The listing builds one solid part. Answer for the finished solid, in the listing's coordinates (mm). A direction names the side the tool comes from. Coordinates: 2 decimals unless noted, no trailing zeros. Loops run counter-clockwise (first coordinate to the right, second up) from the corner with the lowest first, then second, coordinate; pieces in that order, holes last. Notation, with made-up numbers: (3.25, 81.5) - (7.25, 81.5) arc R21 cw to (7.25, 107.5) - close; hole circle Ø3 at (71.5, -23). An arc over 180 degrees is marked (long way). One line per question, with ' | ' between items.
from build123d import *

# Parameters (mm, degrees)
BOSS_EXTRUDE1_DEPTH  = 30
BOSS_EXTRUDE2_START  = -15
BOSS_EXTRUDE2_DEPTH  = 15
CUT_EXTRUDE1_START   = -15
CUT_EXTRUDE1_DEPTH   = 15
SKETCH5_R            = 1.5
CUT_EXTRUDE2_DEPTH   = 15
SKETCH6_R            = 3.1
CUT_EXTRUDE3_DEPTH   = 5
SKETCH7_R            = 1.5
CUT_EXTRUDE4_DEPTH   = 15
SKETCH8_R            = 3.1
CUT_EXTRUDE5_DEPTH   = 5
SKETCH11_R           = 7.5
CUT_EXTRUDE6_DEPTH   = 30
SKETCH12_R           = 11
CUT_EXTRUDE7_DEPTH   = 20
SKETCH13_R           = 4
BOSS_EXTRUDE3_DEPTH  = 20
FILLET1_R            = 2
FILLET1_OF_MIRROR1_R = 2
SKETCH14_R           = 4
CUT_EXTRUDE8_DEPTH   = 40


with BuildPart() as part:
    # Sketch2 → Boss-Extrude1 (new body)
    with BuildSketch(Plane(origin=(0, 0, 0), x_dir=(1, 0, 0), z_dir=(0, 1, 0))):
        with BuildLine():
            Line((-105, 0), (-80, 0))
            ThreePointArc((-80, 0), (0, -80), (80, 0))
            Line((80, 0), (105, 0))
            ThreePointArc((105, 0), (0, -105), (-105, 0))
        make_face()
    extrude(amount=BOSS_EXTRUDE1_DEPTH)

    # Sketch3 → Boss-Extrude2 (add)
    with BuildSketch(Plane(origin=(0, 30, 0), x_dir=(1, 0, 0), z_dir=(0, 1, 0)).offset(BOSS_EXTRUDE2_START)):
        with BuildLine():
            Line((-98.667725183, 35.912115049), (-75.175409663, 27.361611466))
            ThreePointArc((-75.175409663, 27.361611466), (-78.784620241, 13.891854213), (-80, 0))
            Line((-80, 0), (-105, 0))
            ThreePointArc((-105, 0), (-103.404814066, 18.233058655), (-98.667725183, 35.912115049))
        make_face()
    extrude(amount=BOSS_EXTRUDE2_DEPTH)

    # Sketch4 → Cut-Extrude1 (cut)
    with BuildSketch(Plane(origin=(0, 30, 0), x_dir=(1, 0, 0), z_dir=(0, 1, 0)).offset(CUT_EXTRUDE1_START)):
        with BuildLine():
            Line((80, 0), (105, 0))
            ThreePointArc((105, 0), (103.404814066, -18.233058655), (98.667725183, -35.912115049))
            Line((98.667725183, -35.912115049), (75.175409663, -27.361611466))
            ThreePointArc((75.175409663, -27.361611466), (78.784620241, -13.891854213), (80, 0))
        make_face()
    extrude(amount=CUT_EXTRUDE1_DEPTH, mode=Mode.SUBTRACT)

    # Sketch5 → Cut-Extrude2 (cut)
    with BuildSketch(Plane(origin=(0, 15, 0), x_dir=(1, 0, 0), z_dir=(0, 1, 0))):
        with Locations(Location((91.088089232, -16.1, 0), (0, 0, 270))):
            Circle(SKETCH5_R)
    extrude(amount=-CUT_EXTRUDE2_DEPTH, mode=Mode.SUBTRACT)

    # Sketch6 → Cut-Extrude3 (cut)
    with BuildSketch(Plane(origin=(0, 0, 0), x_dir=(-1, 0, 0), z_dir=(0, -1, 0))):
        with Locations(Location((-91.088089232, -16.1, 0), (0, 0, 90))):
            Circle(SKETCH6_R)
    extrude(amount=-CUT_EXTRUDE3_DEPTH, mode=Mode.SUBTRACT)

    # Sketch7 → Cut-Extrude4 (cut)
    with BuildSketch(Plane.XZ.offset(-15)):
        with Locations(Location((-91.088089232, -16.1, 0), (0, 0, 270))):
            Circle(SKETCH7_R)
    extrude(amount=-CUT_EXTRUDE4_DEPTH, mode=Mode.SUBTRACT)

    # Sketch8 → Cut-Extrude5 (cut)
    with BuildSketch(Plane(origin=(0, 30, 0), x_dir=(1, 0, 0), z_dir=(0, 1, 0))):
        with Locations(Location((-91.088089232, 16.1, 0), (0, 0, 270))):
            Circle(SKETCH8_R)
    extrude(amount=-CUT_EXTRUDE5_DEPTH, mode=Mode.SUBTRACT)

    # Sketch11 → Cut-Extrude6 (cut)
    with BuildSketch(Plane.XY.offset(105)):
        with Locations((0, 15)):
            Circle(SKETCH11_R)
    extrude(amount=-CUT_EXTRUDE6_DEPTH, mode=Mode.SUBTRACT)

    # Sketch12 → Cut-Extrude7 (cut)
    with BuildSketch(Plane.XY.offset(105)):
        with Locations((0, 15)):
            Circle(SKETCH12_R)
    extrude(amount=-CUT_EXTRUDE7_DEPTH, mode=Mode.SUBTRACT)

    # Sketch13 → Boss-Extrude3 (add)
    with BuildSketch(Plane.XZ):
        with Locations(Location((-65.40737726, 65.40737726, 0), (0, 0, 270))):
            Circle(SKETCH13_R)
    boss_extrude3 = extrude(amount=BOSS_EXTRUDE3_DEPTH)

    # Fillet1
    fillet1_edges = [part.edges().sort_by_distance(p)[0] for p in [
        (-65.40737726, -20, 69.40737726),
    ]]
    fillet(fillet1_edges, radius=FILLET1_R)

    # Mirror1: Boss-Extrude3 across plane
    add(boss_extrude3.mirror(Plane(origin=(0, 0, 0), x_dir=(0, 0, 1), z_dir=(1, 0, 0))))

    # Fillet1 of Mirror1
    fillet1_of_mirror1_edges = [part.edges().sort_by_distance(p)[0] for p in [
        (65.40737726, -20, 69.40737726),
    ]]
    fillet(fillet1_of_mirror1_edges, radius=FILLET1_OF_MIRROR1_R)

    # Sketch14 → Cut-Extrude8 (cut)
    with BuildSketch(Plane(origin=(-74.246212025, 0, 74.246212025), x_dir=(0, -1, 0), z_dir=(-0.7071067811865488, 0, 0.7071067811865464))):
        with Locations(Location((-15, 0, 0), (0, 0, 90))):
            Circle(SKETCH14_R)
    extrude(amount=-CUT_EXTRUDE8_DEPTH, mode=Mode.SUBTRACT)


solid = part.part
Item 1: Find section A-A, the plane x = 0. Write down the section's boundary in (y, z), plus the area to 3 significant figures.
Taken from the geometry:
outline: (0, 80) - (7.5, 80) - (7.5, 85) - (4, 85) - (4, 105) - (0, 105) - close; (22.5, 80) - (30, 80) - (30, 105) - (26, 105) - (26, 85) - (22.5, 85) - close | area: 235 mm2
Item 2: The mould has two halves that part along X. Classify faces 6 (the face through (-62.797, 16.201, 68.193)), 7 (the face through (64.21, -8.87, 61.59)), 8 (the face through (-87.1, 22.4, -31.7)), 9 (the face through (-33, 30, 81)): pulls with the +X half, pulls with the -X half, needs draft (parallel to the pull), parting line crosses it, or undercut.
Taken from the geometry:
face 6: undercut | face 7: undercut | face 8: pulls with the +X half | face 9: needs draft
Item 3: Which of the six approach directions +Z, -Z, +X, -X, +Y, -Y give full straight-line access (tool end or side, diameter ignored) to faces 1 (the face through (-92, 25, -18)), 2 (the face through (90, 15, 18)), 3 (the face through (-93, 7, 0)), 4 (the face through (-64.21, -8.87, 61.59)), 5 (the face through (7.2, 17.6, 85))?
Taken from the geometry:
face 1: +Y | face 2: -Z, +X, +Y | face 3: -Z, +X, -X, -Y | face 4: -Y | face 5: +Z
Item 4: Each of these flat-tipped pins is pushed along its axis until it touches: pin 1 Ø9 at (x, z) = (-94.5, -17) entering from -Y; pin 2 Ø5 at (x, y) = (-71, 0) entering from -Z; pin 3 Ø12 at (x, y) = (-90, 6.5) entering from -Z; pin 4 Ø12 at (x, y) = (0, 15) entering from +Z. Where does it stop, or does it pass through?
Taken from the geometry:
pin 1: stops at y = 15 | pin 2: stops at z = 31.59 | pin 3: stops at z = 0 | pin 4: passes through
Item 5: Find section D-D, the plane z = -23. Write down the section's boundary in (x, y), plus the area to 3 significant figures.
Taken from the geometry:
outline: (-102.45, 15) - (-76.62, 15) - (-76.62, 30) - (-102.45, 30) - close | area: 387 mm2
Item 6: Find section B-B, the plane z = 49. Write down the section's boundary in (x, y).
Taken from the geometry:
outline: (-92.87, 0) - (-63.24, 0) - (-63.24, 30) - (-92.87, 30) - close; (63.24, 0) - (92.87, 0) - (92.87, 30) - (63.24, 30) - close
Item 7: Find the intervals of material crossed by line 1 (Y direction, x = 69, z = 79); line 2 (Y direction, x = 0, z = 82.25); line 3 (X direction, y = 25, z = 59), in increasing order. Write a range as [from, to].
Taken from the geometry:
line 1: y = [0, 30] | line 2: y = [0, 7.5], [22.5, 30] | line 3: x = [-86.86, -54.03], [54.03, 86.86]
Item 8: Find section C-C, the plane y = -10. Write down the section's boundary in (x, z).
Taken from the geometry:
outline: circle Ø8 at (-65.41, 65.41); circle Ø8 at (65.41, 65.41)
